Check sheet for the modelled part. Datum: model origin and axes. Units: mm. Give positions to 0.01 mm unless a question says otherwise; leave off trailing zeros. Write each loop counter-clockwise with the first axis right and the second up, starting at its lowest first coordinate (ties: lowest second). Pieces come first, ordered by that corner, then holes. Notation, with made-up numbers: (84, -29.75) -> (116, -29.75) arc R11 cw to (116, -18.75) -> close; hole circle Ø1 at (-26, 21). An arc over 180 degrees is marked (long way). Use a Markdown table: item, result. Add a question column.
1. Scan lines: probe 1 along X at (y, z) = (1.05, -2.5); probe 2 along X at (y, z) = (0.9, -26.5); probe 3 along Z at (x, y) = (14, 0.8). Record each from-to range of solid material in increasing order. Write a range as [from, to].
2. Gauge pin test, flat ends, axial feed: P1, Ø1.8, axis at x = 32, z = -2.5, coming from the -Y side; P2, Ø1.5, axis at y = 2.5, z = -46.5, coming from the +X side; P3, Ø0.9, axis at y = 2, z = -57.5, coming from the -X side. Record the tip position at first contact, or that the pin passes through.
3. Cross-section at C-C (y = 1.8). Enter the section's corners in (x, z).
4. Cross-section at D-D (x = 20). Enter the section's corners in (y, z), then the cut area to 3 significant figures.
5. Cross-section at B-B (z = -12). Enter the section's corners in (x, y), then the cut area to 3 significant figures.
6. Cross-section at A-A (x = 8). Enter the section's corners in (y, z), then the cut area to 4 significant figures.
from build123d import *

# Parameters (mm, degrees)
SKETCH1_W           = 40
SKETCH1_H           = 60
BOSS_EXTRUDE1_DEPTH = 3.05
SKETCH4_W           = 3.3
SKETCH4_H           = 52
SKETCH4_W_2         = 3
SKETCH4_H_2         = 0.8
CUT_EXTRUDE1_DEPTH  = 10
CUT_EXTRUDE3_DEPTH  = 10
SKETCH7_R           = 1.5
CUT_EXTRUDE4_DEPTH  = 10


with BuildPart() as part:
    # Sketch1 → Boss-Extrude1 (new body)
    with BuildSketch(Plane(origin=(0, 0, 0), x_dir=(1, 0, 0), z_dir=(0, 1, 0))):
        with Locations((20, 30)):
            Rectangle(SKETCH1_W, SKETCH1_H)
    extrude(amount=BOSS_EXTRUDE1_DEPTH)

    # Sketch4 → Cut-Extrude1 (cut)
    with BuildSketch(Plane(origin=(0, 3.05, 0), x_dir=(1, 0, 0), z_dir=(0, 1, 0))):
        with Locations((20, 30)):
            Rectangle(SKETCH4_W, SKETCH4_H)
        with Locations((20, 57.6)):
            Rectangle(SKETCH4_W_2, SKETCH4_H_2)
    extrude(amount=-CUT_EXTRUDE1_DEPTH, mode=Mode.SUBTRACT)

    # Sketch6 → Cut-Extrude3 (cut)
    with BuildSketch(Plane(origin=(0, 3.05, 0), x_dir=(1, 0, 0), z_dir=(0, 1, 0))):
        Polygon((0, 60), (0, 45), (15, 60), align=None)
        Polygon((40, 60), (40, 45), (25, 60), align=None)
    extrude(amount=-CUT_EXTRUDE3_DEPTH, mode=Mode.SUBTRACT)

    # Sketch7 → Cut-Extrude4 (cut)
    with BuildSketch(Plane(origin=(0, 3.05, 0), x_dir=(1, 0, 0), z_dir=(0, 1, 0))):
        with Locations(Location((8, 2.5, 0), (0, 0, 270))):
            Circle(SKETCH7_R)
        with Locations(Location((32, 2.5, 0), (0, 0, 270))):
            Circle(SKETCH7_R)
    extrude(amount=-CUT_EXTRUDE4_DEPTH, mode=Mode.SUBTRACT)


solid = part.part
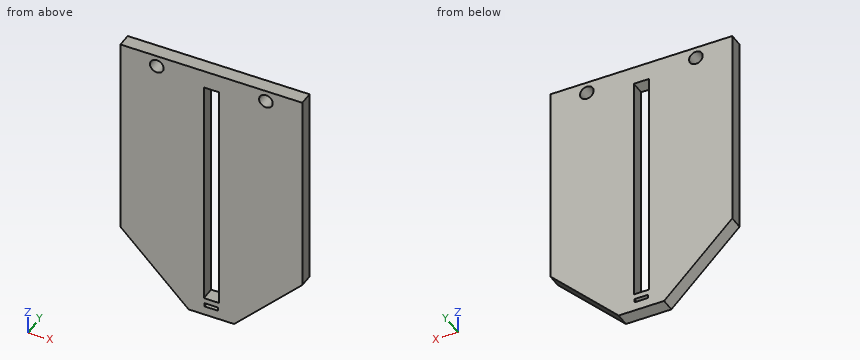
Worked answers:
| question | item | result |
|---|---|---|
| 1 | probe 1 | x = [0, 6.5], [9.5, 30.5], [33.5, 40] |
| 1 | probe 2 | x = [0, 18.35], [21.65, 40] |
| 1 | probe 3 | z = [-59, 0] |
| 2 | P1 | passes through |
| 2 | P2 | stops at x = 39.25 |
| 2 | P3 | stops at x = 12.05 |
| 3 | outline | (0, -45) -> (15, -60) -> (25, -60) -> (40, -45) -> (40, 0) -> (0, 0) -> close; hole circle Ø3 at (8, -2.5); hole (18.35, -56) -> (21.65, -56) -> (21.65, -4) -> (18.35, -4) -> close; hole (18.5, -58) -> (21.5, -58) -> (21.5, -57.2) -> (18.5, -57.2) -> close; hole circle Ø3 at (32, -2.5) |
| 4 | outline | (0, -60) -> (3.05, -60) -> (3.05, -58) -> (0, -58) -> close; (0, -57.2) -> (3.05, -57.2) -> (3.05, -56) -> (0, -56) -> close; (0, -4) -> (3.05, -4) -> (3.05, 0) -> (0, 0) -> close |
| 4 | area | 22.0 mm² |
| 5 | outline | (0, 0) -> (18.35, 0) -> (18.35, 3.05) -> (0, 3.05) -> close; (21.65, 0) -> (40, 0) -> (40, 3.05) -> (21.65, 3.05) -> close |
| 5 | area | 112 mm² |
| 6 | outline | (0, -53) -> (3.05, -53) -> (3.05, -4) -> (0, -4) -> close; (0, -1) -> (3.05, -1) -> (3.05, 0) -> (0, 0) -> close |
| 6 | area | 152.5 mm² |
